from build123d import *

# Parameters (mm, degrees)
F1_DEPTH  = 5
F3_DEPTH  = 10
F5_DEPTH  = 10
F7_DEPTH  = 10
F8_R      = 2.5
F9_DEPTH  = 25.4
F10_R     = 2.5
F11_DEPTH = 25.4
F12_R     = 2.5
F13_DEPTH = 25.4
F15_DEPTH = 30


with BuildPart() as f1:
    # F0 (on Top) → F1 (new body, symmetric)
    with BuildSketch(Plane.XY):
        Polygon((-25, 43.3012701892), (-30, 51.9615242271), (-20, 51.9615242271), (-28.6602540378, 56.9615242271), (-33.6602540378, 48.3012701892), align=None)
        Polygon((-20, 51.9615242271), (-30, 51.9615242271), (-25, 43.3012701892), align=None)
        Polygon((20, 51.9615242271), (-20, 51.9615242271), (-25, 43.3012701892), (-5, 8.6602540378), (5, 8.6602540378), (25, 43.3012701892), align=None)
        Polygon((28.6602540378, 56.9615242271), (20, 51.9615242271), (30, 51.9615242271), (25, 43.3012701892), (33.6602540378, 48.3012701892), align=None)
        Polygon((30, 51.9615242271), (20, 51.9615242271), (25, 43.3012701892), align=None)
        Polygon((5, 8.6602540378), (-5, 8.6602540378), (0, 0), align=None)
        Polygon((0, 0), (-5, 8.6602540378), (-5, -1.3397459622), (5, -1.3397459622), (5, 8.6602540378), align=None)
    extrude(amount=F1_DEPTH, both=True)

    # F2 (on face) → F3 (join)
    with BuildSketch(Plane(origin=(12.5, 21.6506350946, 0), x_dir=(0.8660254038, -0.5, 0), z_dir=(-0.5, -0.8660254038, 0))):
        with BuildLine():
            Line((-53.3012701892, -5), (-53.3012701892, 5))
            ThreePointArc((-53.3012701892, 5), (-58.3012701892, 0), (-53.3012701892, -5))
        make_face()
    extrude(amount=-F3_DEPTH)

    # F4 (on face) → F5 (join)
    with BuildSketch(Plane(origin=(-17.5, 30.3108891325, 0), x_dir=(-0.8660254038, -0.5, 0), z_dir=(-0.5, 0.8660254038, 0))):
        with BuildLine():
            Line((-53.3012701892, -5), (-53.3012701892, 5))
            ThreePointArc((-53.3012701892, 5), (-58.3012701892, 0), (-53.3012701892, -5))
        make_face()
    extrude(amount=-F5_DEPTH)

    # F6 (on face) → F7 (join)
    with BuildSketch(Plane.YZ.offset(5)):
        with BuildLine():
            Line((-1.3397459622, -5), (-1.3397459622, 5))
            ThreePointArc((-1.3397459622, 5), (-6.3397459622, 0), (-1.3397459622, -5))
        make_face()
    extrude(amount=-F7_DEPTH)

    # F8 (on face) → F9 (cut)
    with BuildSketch(Plane.YZ.offset(5)):
        with Locations((-1.3397459622, 0)):
            Circle(F8_R)
    extrude(amount=-F9_DEPTH, mode=Mode.SUBTRACT)

    # F10 (on face) → F11 (cut)
    with BuildSketch(Plane(origin=(-17.5, 30.3108891325, 0), x_dir=(-0.8660254038, -0.5, 0), z_dir=(-0.5, 0.8660254038, 0))):
        with Locations((-53.3012701892, 0)):
            Circle(F10_R)
    extrude(amount=-F11_DEPTH, mode=Mode.SUBTRACT)

    # F12 (on face) → F13 (cut)
    with BuildSketch(Plane(origin=(12.5, 21.6506350946, 0), x_dir=(0.8660254038, -0.5, 0), z_dir=(-0.5, -0.8660254038, 0))):
        with Locations((-53.3012701892, 0)):
            Circle(F12_R)
    extrude(amount=-F13_DEPTH, mode=Mode.SUBTRACT)

    # F14 (on face) → F15 (join)
    with BuildSketch(Plane(origin=(0, 0, -5), x_dir=(1, 0, 0), z_dir=(0, 0, -1))):
        with BuildLine():
            ThreePointArc((-12.9903810568, -42.1410161514), (-7.5, -47.6313972081), (0, -49.6410161514))
            Line((0, -49.6410161514), (0, -46.6410161514))
            ThreePointArc((0, -46.6410161514), (-6, -45.0333209968), (-10.3923048454, -40.6410161514))
            Line((-10.3923048454, -40.6410161514), (-12.9903810568, -42.1410161514))
        make_face()
        with BuildLine():
            Line((0, -46.6410161514), (0, -49.6410161514))
            ThreePointArc((0, -49.6410161514), (7.5, -47.6313972081), (12.9903810568, -42.1410161514))
            Line((12.9903810568, -42.1410161514), (10.3923048454, -40.6410161514))
            ThreePointArc((10.3923048454, -40.6410161514), (6, -45.0333209968), (0, -46.6410161514))
        make_face()
        with BuildLine():
            ThreePointArc((-12.9903810568, -27.1410161514), (-15, -34.6410161514), (-12.9903810568, -42.1410161514))
            Line((-12.9903810568, -42.1410161514), (-10.3923048454, -40.6410161514))
            ThreePointArc((-10.3923048454, -40.6410161514), (-12, -34.6410161514), (-10.3923048454, -28.6410161514))
            Line((-10.3923048454, -28.6410161514), (-12.9903810568, -27.1410161514))
        make_face()
        with BuildLine():
            Line((10.3923048454, -40.6410161514), (12.9903810568, -42.1410161514))
            ThreePointArc((12.9903810568, -42.1410161514), (14.4888873943, -38.5233018279), (15, -34.6410161514))
            ThreePointArc((15, -34.6410161514), (14.4888873943, -30.7587304748), (12.9903810568, -27.1410161514))
            Line((12.9903810568, -27.1410161514), (10.3923048454, -28.6410161514))
            ThreePointArc((10.3923048454, -28.6410161514), (11.5911099155, -31.5351876101), (12, -34.6410161514))
            ThreePointArc((12, -34.6410161514), (11.5911099155, -37.7468446926), (10.3923048454, -40.6410161514))
        make_face()
        with BuildLine():
            ThreePointArc((0, -19.6410161514), (-7.5, -21.6506350946), (-12.9903810568, -27.1410161514))
            Line((-12.9903810568, -27.1410161514), (-10.3923048454, -28.6410161514))
            ThreePointArc((-10.3923048454, -28.6410161514), (-6, -24.248711306), (0, -22.6410161514))
            Line((0, -22.6410161514), (0, -19.6410161514))
        make_face()
        with BuildLine():
            Line((0, -19.6410161514), (0, -22.6410161514))
            ThreePointArc((0, -22.6410161514), (6, -24.248711306), (10.3923048454, -28.6410161514))
            Line((10.3923048454, -28.6410161514), (12.9903810568, -27.1410161514))
            ThreePointArc((12.9903810568, -27.1410161514), (7.5, -21.6506350946), (0, -19.6410161514))
        make_face()
    extrude(amount=F15_DEPTH)


solid = f1.part
The listing builds one solid part. Answer for the finished solid, in the listing's coordinates (mm). A direction names the side the tool comes from. Coordinates: 2 decimals unless noted, no trailing zeros. Order: outer loops, then holes, each group sorted by start corner. A loop starts at its lowest first (then second) coordinate and runs counter-clockwise, first axis right, second up. Notation, with made-up numbers: (54, 3.5) -> (113, 3.5) arc R13 cw to (113, 14.5) -> close; hole circle Ø3 at (-7.75, -20.5). An arc over 180 degrees is marked (long way). Answer in a Markdown table with one row per item. Add a question column.
Item 1: Find section D-D (z = 0). Write down the section's boundary in (x, y).
Item 2: Each of these flat-tipped pins is pushed along its axis until it touches: P1, Ø3, axis at x = 18.5, y = 51, coming from the -Z side; P2, Ø6, axis at y = 41.5, z = -9, coming from the +X side; P3, Ø4, axis at y = -1.34, z = 0, coming from the +X side; P4, Ø11, axis at y = 1, z = -0.5, coming from the +X side. Where does it stop, or does it pass through?
Item 3: Find section A-A (z = -27). Write down the section's boundary in (x, y).
Item 4: Find the intervals of material crossed by L1, parallel to X at y = 50.5, z = -0.5; L2, parallel to X at y = 35, z = -20; L3, parallel to X at y = 32.5, z = -27, in increasing order. Write a range as from..to.
Item 5: Which of the six approach directions +Z, -Z, +X, -X, +Y, -Y give full straight-line access (tool end or side, diameter ignored) to faces 4 (the face through (5, 3, 0)), 5 (the face through (2, 50, -5)), 6 (the face through (0, 51.962, 0))?
Item 6: Find section B-B (x = 2.5). Write down the section's boundary in (y, z).
Item 7: Determine the mould class of faces 1 (the face through (14.86, 25.74, 0.07)), 2 (the face through (0, 35, -5)), 3 (the face through (35.454, 55.191, 0.11)) for opening direction Y: +Y half, -Y half, draft (parallel to the pull), parting line (faces both ways), or undercut.
Item 8: Find section C-C (y = 37.5). Write down the section's boundary in (x, z), then the cut area to 3 significant figures.
Result set:
| question | item | result |
|---|---|---|
| 1 | outline | (-37.99, 50.8) -> (-35.83, 49.55) -> (-30.83, 58.21) -> (-32.99, 59.46) -> close; (-31.5, 47.05) -> (-25, 43.3) -> (-5, 8.66) -> (-5, 1.16) -> (5, 1.16) -> (5, 8.66) -> (25, 43.3) -> (31.5, 47.05) -> (26.5, 55.71) -> (20, 51.96) -> (-20, 51.96) -> (-26.5, 55.71) -> close; (-5, -6.34) -> (5, -6.34) -> (5, -3.84) -> (-5, -3.84) -> close; (30.83, 58.21) -> (35.83, 49.55) -> (37.99, 50.8) -> (32.99, 59.46) -> close |
| 2 | P1 | stops at z = -5 |
| 2 | P2 | stops at x = 14.5 |
| 2 | P3 | passes through |
| 2 | P4 | stops at x = 5 |
| 3 | outline | circle Ø30 at (0, 34.64); hole circle Ø24 at (0, 34.64) |
| 4 | L1 | x = -37.47..-35.22, -29.56..29.56, 35.22..37.47 |
| 4 | L2 | x = -15..-11.99, 11.99..15 |
| 4 | L3 | x = -14.85..-11.81, 11.81..14.85 |
| 5 | face 4 | +Z, -Z, +X, -Y |
| 5 | face 5 | -Z |
| 5 | face 6 | +Z, -Z, +Y |
| 6 | outline | (-1.34, -5) -> (19.85, -5) -> (19.85, -35) -> (22.9, -35) -> (22.9, -5) -> (46.38, -5) -> (46.38, -35) -> (49.43, -35) -> (49.43, -5) -> (51.96, -5) -> (51.96, 5) -> (-1.34, 5) arc R5 ccw to start; hole circle Ø5 at (-1.34, 0) |
| 7 | face 1 | -Y half |
| 7 | face 2 | undercut |
| 7 | face 3 | +Y half |
| 8 | outline | (-21.65, -5) -> (-14.73, -5) -> (-14.73, -35) -> (-11.65, -35) -> (-11.65, -5) -> (11.65, -5) -> (11.65, -35) -> (14.73, -35) -> (14.73, -5) -> (21.65, -5) -> (21.65, 5) -> (-21.65, 5) -> close |
| 8 | area | 617 mm² |
